Check sheet for the modelled part. Datum: model origin and axes. Units: mm. Give positions to 0.01 mm unless a question says otherwise; leave off trailing zeros. Loops run counter-clockwise (first coordinate to the right, second up) from the corner with the lowest first, then second, coordinate; pieces in that order, holes last.
```python
from build123d import *

# Parameters (mm, degrees)
SKETCH1_R            = 335
SKETCH1_R_2          = 295
BOSS_EXTRUDE1_DEPTH  = 10
BOSS_EXTRUDE2_DEPTH  = 10
BOSS_EXTRUDE3_DEPTH  = 10
CUT_EXTRUDE1_DEPTH   = 10
CUT_EXTRUDE2_START   = 272.424930167
CUT_EXTRUDE2_DEPTH   = 38.548591659
CUT_EXTRUDE2_START_2 = 161.824552733
CUT_EXTRUDE2_2_DEPTH = 10
BOSS_EXTRUDE4_DEPTH  = 10


with BuildPart() as part:
    # Sketch1 → Boss-Extrude1 (new body)
    with BuildSketch(Plane.XY):
        Circle(SKETCH1_R)
        Circle(SKETCH1_R_2, mode=Mode.SUBTRACT)
    extrude(amount=BOSS_EXTRUDE1_DEPTH)

    # Sketch2 → Boss-Extrude2 (add)
    with BuildSketch(Plane(origin=(0, 0, 0), x_dir=(-1, 0, 0), z_dir=(0, 0, -1))):
        with BuildLine():
            ThreePointArc((-322.474278085, 90.748773952), (-285.195118694, 175.7519396), (-226.022138309, 247.263003691))
            Line((-226.022138309, 247.263003691), (-312.556910604, 168.161908985))
            ThreePointArc((-312.556910604, 168.161908985), (-313.727388299, 166.889496734), (-314.661210657, 165.434496124))
            ThreePointArc((-314.661210657, 165.434496124), (-328.310849458, 136.353350264), (-339.27949001, 106.158738023))
            ThreePointArc((-339.27949001, 106.158738023), (-338.523562212, 98.412053492), (-332.442347906, 93.553928275))
            Line((-332.442347906, 93.553928275), (-322.474278085, 90.748773952))
        make_face()
    extrude(amount=-BOSS_EXTRUDE2_DEPTH)

    # Sketch3 → Boss-Extrude3 (add)
    with BuildSketch(Plane(origin=(0, 0, 0), x_dir=(-1, 0, 0), z_dir=(0, 0, -1))):
        with BuildLine():
            Line((-289.450839465, -149.430532958), (-290.086949825, -136.323752762))
            Line((-290.086949825, -136.323752762), (-321.966145398, -92.535405211))
            Line((-321.966145398, -92.535405211), (-332.178557921, -95.470526635))
            ThreePointArc((-332.178557921, -95.470526635), (-338.234587628, -100.365745681), (-338.943329669, -108.120508737))
            ThreePointArc((-338.943329669, -108.120508737), (-327.253686464, -139.562351058), (-312.654741, -169.763476834))
            Line((-312.654741, -169.763476834), (-223.394344885, -249.639673677))
            Line((-223.394344885, -249.639673677), (-289.450839465, -149.430532958))
        make_face()
    extrude(amount=-BOSS_EXTRUDE3_DEPTH)

    # Sketch4 → Cut-Extrude1 (cut)
    with BuildSketch(Plane(origin=(23.906119202, -116.35832345, 93.20136559), x_dir=(0.9873859847265816, 0.12357681316719145, -0.0989832733999036), z_dir=(-0.15833166823323438, 0.7706481888305408, -0.6172782613106412))):
        Polygon((282.331330651, 83.607742228), (286.950805192, 120.032776555), (337.459038649, 113.627250716), (329.847523561, 53.609667359), (279.339290104, 60.015193198), align=None)
    extrude(amount=-CUT_EXTRUDE1_DEPTH, mode=Mode.SUBTRACT)

    # Cut-Extrude2: read off the stored shape, not the designer's step
    # Cut-Extrude2 outline → Cut-Extrude2 (cut)
    with BuildSketch(Plane(origin=(0, 0, 0), x_dir=(0.20124905404319107, 0.9795401054815064, 0), z_dir=(0.9795401054815065, -0.20124905404319107, 0)).offset(CUT_EXTRUDE2_START)):
        Polygon((202.006915017, 0), (195.824910476, 10), (184.068330185, 10), (190.250334726, 0), align=None)
    extrude(amount=CUT_EXTRUDE2_DEPTH, mode=Mode.SUBTRACT)

    # Cut-Extrude2 2 outline → Cut-Extrude2 2 (cut)
    with BuildSketch(Plane(origin=(0, 0, 0), x_dir=(0.9852397845422891, -0.14476117541924635, -0.09136065370990885), z_dir=(0.1711799256778192, 0.8331845496216821, 0.5258335661753164)).offset(CUT_EXTRUDE2_START_2)):
        with BuildLine():
            Line((280.153711914, 76.574004203), (278.423879054, 60.562054707))
            add(Edge.make_bspline(
                [(278.423879054, 60.562054707), (279.04318666, 59.849827211), (279.679221342, 59.165584066), (280.331358402, 58.511847756)],
                knots=[0.202262646, 0.202262646, 0.202262646, 0.202262646, 0.204525626, 0.204525626, 0.204525626, 0.204525626], degree=3))
            Line((280.331358402, 58.511847756), (282.258121917, 76.346656647))
            Line((282.258121917, 76.346656647), (282.436738997, 78))
            Line((282.436738997, 78), (280.307767758, 78))
            Line((280.307767758, 78), (280.153711914, 76.574004203))
        make_face()
    extrude(amount=CUT_EXTRUDE2_2_DEPTH, mode=Mode.SUBTRACT)

    # Sketch6 → Boss-Extrude4 (add)
    with BuildSketch(Plane(origin=(0, 0, 0), x_dir=(-1, 0, 0), z_dir=(0, 0, -1))):
        with BuildLine():
            Line((297.863422842, -159.420809844), (324.396421164, -145.420809844))
            ThreePointArc((324.396421164, -145.420809844), (328.498305309, -135.901116291), (332.320896217, -126.265877963))
            ThreePointArc((332.320896217, -126.265877963), (332.034149526, -118.483971626), (326.252641154, -113.267224475))
            Line((326.252641154, -113.267224475), (309.887866806, -107.585760677))
            Line((309.887866806, -107.585760677), (279.768360506, -168.96857635))
            Line((279.768360506, -168.96857635), (279.768360506, -180.275251772))
            Line((279.768360506, -180.275251772), (256.883838664, -211.365229457))
            Line((256.883838664, -211.365229457), (299.577700502, -188.838033003))
            ThreePointArc((299.577700502, -188.838033003), (301.757845667, -187.282127202), (303.446809055, -185.203358702))
            ThreePointArc((303.446809055, -185.203358702), (310.564518318, -173.00268773), (317.191935305, -160.528895148))
            Line((317.191935305, -160.528895148), (302.530089508, -168.265142618))
            Line((302.530089508, -168.265142618), (297.863422842, -159.420809844))
        make_face()
        with BuildLine():
            Line((324.396421164, 145.420809844), (297.863422842, 159.420809844))
            Line((297.863422842, 159.420809844), (302.530089508, 168.265142618))
            Line((302.530089508, 168.265142618), (317.191935305, 160.528895148))
            ThreePointArc((317.191935305, 160.528895148), (310.564518318, 173.00268773), (303.446809055, 185.203358702))
            ThreePointArc((303.446809055, 185.203358702), (301.757845667, 187.282127202), (299.577700502, 188.838033003))
            Line((299.577700502, 188.838033003), (256.883838664, 211.365229457))
            Line((256.883838664, 211.365229457), (279.768360506, 180.275251772))
            Line((279.768360506, 180.275251772), (279.768360506, 168.96857635))
            Line((279.768360506, 168.96857635), (309.887866806, 107.585760677))
            Line((309.887866806, 107.585760677), (326.252641154, 113.267224475))
            ThreePointArc((326.252641154, 113.267224475), (332.034149526, 118.483971626), (332.320896217, 126.265877963))
            ThreePointArc((332.320896217, 126.265877963), (328.498305309, 135.901116291), (324.396421164, 145.420809844))
        make_face()
    extrude(amount=-BOSS_EXTRUDE4_DEPTH)


solid = part.part
```
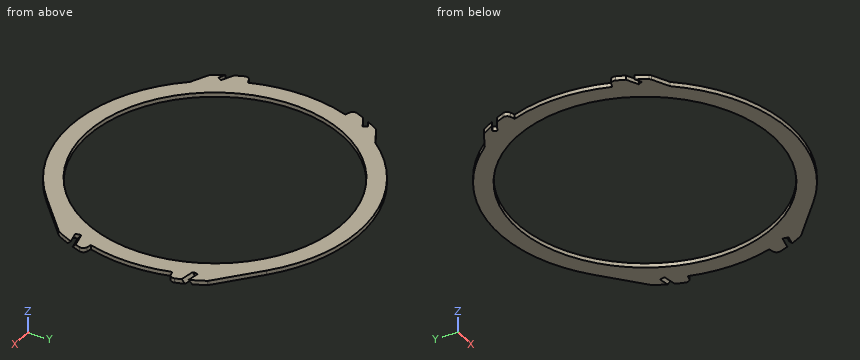
(1) Gauge pin test, flat ends, axial feed: pin 1 Ø3 at (y, z) = (138, 3.5) entering from +X; pin 2 Ø3 at (x, z) = (183.5, 1.5) entering from -Y; pin 3 Ø5 at (y, z) = (-196, 4.5) entering from -X. Record the tip position at first contact, or that the pin passes through.
(2) Section check B-B on x = -180. Record the boundary of the cut face in (y, z), plus the area to 3 significant figures.
(3) Material ranges on line 1 (Y direction, x = 0, z = 6); line 2 (X direction, y = 164, z = 2.75); line 3 (Y direction, x = 164, z = 8.5), recorded low to high.
(4) Section check A-A on y = 0. Record the boundary of the cut face in (x, z), plus the area to 3 significant figures.
Computed values:
1. pin 1: stops at x = 328.25
1. pin 2: stops at y = -281.25
1. pin 3: stops at x = -290.74
2. outline: (-282.53, 0) - (-233.72, 0) - (-233.72, 10) - (-282.53, 10) - close; (233.72, 0) - (282.53, 0) - (282.53, 10) - (233.72, 10) - close
2. area: 976 mm2
3. line 1: y = -335 to -295, 295 to 335
3. line 2: x = -315.41 to -310.61, -300.28 to -245.21, 245.21 to 315.41
3. line 3: y = -292.11 to -245.21, 245.21 to 292.11
4. outline: (-335, 0) - (-295, 0) - (-295, 10) - (-335, 10) - close; (295, 0) - (335, 0) - (335, 10) - (295, 10) - close
4. area: 800 mm2
